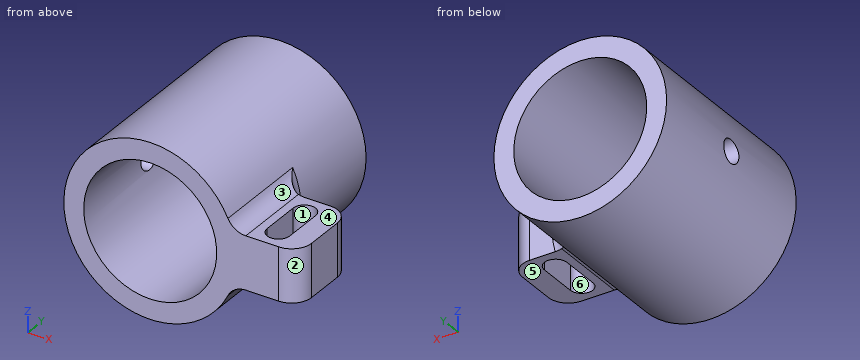
from build123d import *

# Parameters (mm, degrees)
SKETCH_1_R             = 13.05
SKETCH_1_R_2           = 10.05
EXTRUDE_1_DEPTH        = 15
EXTRUDE_2_REACH        = 35.782
EXTRUDE_2_START_RADIUS = 13.05
EXTRUDE_2_END_RADIUS   = 13.05
SKETCH_2_W             = 8
SKETCH_2_H             = 12
CUT_EXTRUDE_1_DEPTH    = 33.025068306
CUT_EXTRUDE_2_DEPTH    = 32.913039886
FILLET_1_R             = 3
FILLET_2_R             = 3
SKETCH_6_R             = 1.75
CUT_EXTRUDE_3_DEPTH    = 30.967350938


with BuildPart() as part:
    # 草图1 → 凸台-拉伸1 (new, symmetric)
    with BuildSketch(Plane(origin=(0, 0, 0), x_dir=(1, 0, 0), z_dir=(0, 1, 0))):
        with Locations(Location((0, 0, 0), (0, 0, 270))):
            Circle(SKETCH_1_R)
        with Locations(Location((0, 0, 0), (0, 0, 270))):
            Circle(SKETCH_1_R_2, mode=Mode.SUBTRACT)
    extrude(amount=EXTRUDE_1_DEPTH, both=True)

    # 凸台-拉伸2: from a cylinder face, 35.782 long prism both ways, kept between that surface and its translate by the depth
    extrude_2_start = Plane(origin=(0, -9, 0), z_dir=(0, -1, 0)) * Cylinder(EXTRUDE_2_START_RADIUS, 98.664, mode=Mode.PRIVATE)
    extrude_2_end = Plane(origin=(10, -9, 0), z_dir=(0, -1, 0)) * Cylinder(EXTRUDE_2_END_RADIUS, 98.664, mode=Mode.PRIVATE)
    # 草图2 → 凸台-拉伸2 (add, from a surface)
    with BuildSketch(Plane(origin=(0, 0, 0), x_dir=(0, 0, -1), z_dir=(1, 0, 0)), mode=Mode.PRIVATE) as extrude_2_sk1:
        with Locations((0, -9)):
            Rectangle(SKETCH_2_W, SKETCH_2_H)
    extrude_2_tool1 = extrude(extrude_2_sk1.sketch, amount=EXTRUDE_2_REACH, both=True, mode=Mode.PRIVATE)
    add(((extrude_2_tool1 - extrude_2_start) & extrude_2_end).solids().sort_by_distance((17.421856, -9, 0))[0])

    # 草图4 → 切除-拉伸1 (cut, through all)
    with BuildSketch(Plane(origin=(0, -3, 0), x_dir=(1, 0, 0), z_dir=(0, 1, 0))):
        with BuildLine():
            Line((22.421855739, 4), (22.421855739, -4))
            ThreePointArc((22.421855739, -4), (23.05, 0), (22.421855739, 4))
        make_face()
    extrude(amount=-CUT_EXTRUDE_1_DEPTH, mode=Mode.SUBTRACT)

    # 草图5 → 切除-拉伸2 (cut, through all)
    with BuildSketch(Plane.XY.offset(4)):
        with BuildLine():
            Line((15.721855739, -12), (15.721855739, -6))
            ThreePointArc((15.721855739, -6), (17.421855739, -4.3), (19.121855739, -6))
            Line((19.121855739, -6), (19.121855739, -12))
            ThreePointArc((19.121855739, -12), (17.421855739, -13.7), (15.721855739, -12))
        make_face()
    extrude(amount=-CUT_EXTRUDE_2_DEPTH, mode=Mode.SUBTRACT)

    # 圆角1
    fillet_1_edges = [part.edges().sort_by_distance(p)[0] for p in [
        (22.421855739, -15, 0),
        (22.421855739, -3, 0),
    ]]
    fillet(fillet_1_edges, radius=FILLET_1_R)

    # 圆角2
    fillet_2_edges = [part.edges().sort_by_distance(p)[0] for p in [
        (12.421855739, -9, -4),
        (13.05, -3, 0),
        (12.421855739, -9, 4),
    ]]
    fillet(fillet_2_edges, radius=FILLET_2_R)

    # 草图6 → 切除-拉伸3 (cut, through all)
    with BuildSketch(Plane(origin=(0, 0, 0), x_dir=(0, 0, -1), z_dir=(1, 0, 0))):
        Circle(SKETCH_6_R)
    extrude(amount=-CUT_EXTRUDE_3_DEPTH, mode=Mode.SUBTRACT)


solid = part.part
Can you work these out from the model? Positions are in its coordinate system, mm. Face numbers are marked on the shaded views. A direction names the side the tool comes from. Coordinates: 2 decimals unless noted, no trailing zeros. Loops run counter-clockwise (first coordinate to the right, second up) from the corner with the lowest first, then second, coordinate; pieces in that order, holes last. Notation, with made-up numbers: M 8.5,46.5 L 59.5,46.5 A20 cw 59.5,71.5 Z; hole C -10,-36.5 d9. An arc over 180 degrees is marked long. Return JSON: item names as keys, results as strings. Group by question number.
Item 1: Imagine slicing it at C-C (z = -7.75). Please give me the cut outline in (x, y), and give its area (3 significant figures).
Item 2: On a 3-axis mill with a long thin cutter (end or side, diameter ignored), from which of +Z, -Z, +X, -X, +Y, -Y can I reach the whole of each face in a straight line? I mean the marked faces 4, 5 and 6. Say none if no direction works.
Item 3: Imagine slicing it at A-A (y = -6.5). Please give me the cut outline in (x, z), and give its area (3 significant figures).
Item 4: I'm going to push flat-ended pins straight in: pin 1 Ø2 at (x, y) = (-7.5, -8.5) entering from +Z; pin 2 Ø4 at (y, z) = (-3.5, 1) entering from +X; pin 3 Ø8 at (y, z) = (3, -8.5) entering from -X. Where does each tip first touch, or does it pass through?
Item 5: Imagine slicing it at D-D (z = 3.5). Give the number of separate pieces and of enclosed holes in the cut face, and give its area (3 significant figures).
Item 6: Thinking about a two-plate mould opening in Y: for the marked faces 1, 2 and 3, which applies, released by +Y, released by -Y, zero draft, split by the parting line, or undercut?
Item 7: If I drill on L1, parallel to Y at x = -11.4, z = 0; L2, parallel to X at y = 8.5, z = 0; L3, parallel to Z at x = -3.5, y = 7, over which ranges is the centre line in solid material (lowest first)? Write a range as from..to.
Item 8: Imagine slicing it at B-B (x = 0). Please give me the cut outline in (y, z).
Verdict:
{
 "1": {"outline": "M -10.5,-15 L -6.4,-15 L -6.4,15 L -10.5,15 Z; M 6.4,-15 L 10.5,-15 L 10.5,15 L 6.4,15 Z", "area": "246 mm^2"},
 "2": {"face 4": "+Z, +X, +Y, -Y", "face 5": "-Z, +X, +Y, -Y", "face 6": "+Z, -Z"},
 "3": {"outline": "M 11.74,-5.69 A3 cw 14.44,-4 L 15.72,-4 L 15.72,4 L 14.44,4 A3 cw 11.74,5.69 A13.05 ccw long Z; M 19.12,-4 L 22.42,-4 L 22.42,4 L 19.12,4 Z; hole C 0,0 d20.1", "area": "269 mm^2"},
 "4": {"pin 1": "stops at z = 11.32", "pin 2": "stops at x = 22.38", "pin 3": "stops at x = -12.25"},
 "5": {"separate pieces": "2", "enclosed holes": "1", "area": "276 mm^2"},
 "6": {"face 1": "undercut", "face 2": "released by -Y", "face 3": "zero draft"},
 "7": {"L1": "y = -15..-1.75, 1.75..15", "L2": "x = -13.05..-10.05, 10.05..13.05", "L3": "z = -12.57..-9.42, 9.42..12.57"},
 "8": {"outline": "M -15,-13.05 L 15,-13.05 L 15,-10.05 L -15,-10.05 Z; M -15,10.05 L 15,10.05 L 15,13.05 L -15,13.05 Z"}
}
